```python
from build123d import *

# Parameters (mm, degrees)
SKETCH_1_R      = 1.6
SKETCH_1_R_2    = 7.25
EXTRUDE_1_DEPTH = 2
SKETCH_2_W      = 32.15
SKETCH_2_H      = 18.7
SKETCH_2_R      = 1.6
EXTRUDE_2_DEPTH = 2
FILLET_1_R      = 12
FILLET_2_R      = 1


with BuildPart() as part:
    # 草图1 → 凸台-拉伸1 (new body)
    with BuildSketch(Plane(origin=(0, 0, 0), x_dir=(1, 0, 0), z_dir=(0, 1, 0))):
        with BuildLine():
            Line((0, 0), (64.3, 0))
            Line((64.3, 0), (64.3, 30.6))
            ThreePointArc((64.3, 30.6), (60.521677477, 39.721677477), (51.4, 43.5))
            Line((51.4, 43.5), (12.9, 43.5))
            ThreePointArc((12.9, 43.5), (3.778322523, 39.721677477), (0, 30.6))
            Line((0, 30.6), (0, 0))
        make_face()
        with Locations(Location((7.89764523, 11.4, 0), (0, 0, 270))):
            Circle(SKETCH_1_R, mode=Mode.SUBTRACT)
        with Locations(Location((7.89764523, 37.8, 0), (0, 0, 270))):
            Circle(SKETCH_1_R, mode=Mode.SUBTRACT)
        with Locations(Location((12.9, 24.6, 0), (0, 0, 270))):
            Circle(SKETCH_1_R_2, mode=Mode.SUBTRACT)
        with Locations(Location((56.40235477, 11.4, 0), (0, 0, 90))):
            Circle(SKETCH_1_R, mode=Mode.SUBTRACT)
        with Locations(Location((56.40235477, 37.8, 0), (0, 0, 90))):
            Circle(SKETCH_1_R, mode=Mode.SUBTRACT)
        with Locations(Location((51.4, 24.6, 0), (0, 0, 90))):
            Circle(SKETCH_1_R_2, mode=Mode.SUBTRACT)
    extrude(amount=EXTRUDE_1_DEPTH)

    # 草图2 → 凸台-拉伸2 (add)
    # profile 1 of 2: a face of its own
    with BuildSketch(Plane.XY):
        with Locations((16.075, 11.35)):
            Rectangle(SKETCH_2_W, SKETCH_2_H)
        with Locations((3.15, 9.2)):
            Circle(SKETCH_2_R, mode=Mode.SUBTRACT)
        with Locations((17.15, 17.2)):
            Circle(SKETCH_2_R, mode=Mode.SUBTRACT)
    # profile 2 of 2: a face of its own
    with BuildSketch(Plane.XY):
        with Locations((48.225, 11.35)):
            Rectangle(SKETCH_2_W, SKETCH_2_H)
        with Locations((61.15, 9.2)):
            Circle(SKETCH_2_R, mode=Mode.SUBTRACT)
        with Locations((47.15, 17.2)):
            Circle(SKETCH_2_R, mode=Mode.SUBTRACT)
    extrude(amount=-EXTRUDE_2_DEPTH)

    # 圆角1
    fillet_1_edges = [part.edges().sort_by_distance(p)[0] for p in [
        (0, 20.7, -1),
        (64.3, 20.7, -1),
    ]]
    fillet(fillet_1_edges, radius=FILLET_1_R)

    # 圆角2
    fillet_2_edges = [part.edges().sort_by_distance(p)[0] for p in [
        (32.15, 2, -2),
        (32.15, 0, 0),
    ]]
    fillet(fillet_2_edges, radius=FILLET_2_R)


solid = part.part
```
Part model, mm, in its own coordinate system. A direction names the side the tool comes from. Round coordinates to 2 decimals unless told otherwise and drop trailing zeros. Write each loop counter-clockwise with the first axis right and the second up, starting at its lowest first coordinate (ties: lowest second). Pieces come first, ordered by that corner, then holes. Notation, with made-up numbers: M -10,-15.5 L -5,-15.5 A4 ccw -5,-9.5 Z; hole C 55.25,-34.75 d11. An arc over 180 degrees is marked long. Answer as CSV lines item,"result". Start each with the question number.
1) Mould opens along Z. For faces 3 (the face through (59.55, 9.27, -0.99)), 4 (the face through (32, 1, -43.5)), 5 (the face through (54.816, 0.986, -11.192)), 6 (the face through (7.97, 0.99, -39.4)) say: +Z half, -Z half, draft (parallel to the pull), parting line (faces both ways), or undercut.
2) Band-saw the part on B-B (x = 50). List the corners of the cut face in (y, z), then the cut area to 3 significant figures.
3) Band-saw the part on C-C (x = 17.15). List the corners of the cut face in (y, z), then the cut area to 3 significant figures.
4) Drop flat-ended pins along their axis: pin 1 (5 mm diameter, centred on x = 7.9, z = -11.4, fed in from +Y); pin 2 (3.5 mm diameter, centred on x = 17.15, y = 17.2, fed in from -Z). Give the stop position or say it passes through.
5) Which spindle directions (+Z, -Z, +X, -X, +Y, -Y) get a long thin tool onto all of the face, cutting with end or side? Do faces 1 (the face through (32, 12, -2)), 2 (the face through (3.42, 17.09, -1.01)). Say none if no direction does.
6) Band-saw the part on D-D (x = 39). List the corners of the cut face in (y, z), then the cut area to 3 significant figures.
7) Band-saw the part on A-A (z = -24.6). List the corners of the cut face in (x, y), then the cut area to 3 significant figures.
8) Drill centre lines: L1, parallel to X at y = 0.7, z = -24.6; L2, parallel to Y at x = 43.5, z = -9; L3, parallel to Z at x = 32, y = 13.5. Where is each one in solid material? Low to high.
Worked out:
1,face 3,"draft"
1,face 4,"-Z half"
1,face 5,"undercut"
1,face 6,"undercut"
2,outline,"M 0,-43.5 L 2,-43.5 L 2,-31.71 L 0,-31.71 Z; M 0,-17.49 L 2,-17.49 L 2,-3 A1 cw 3,-2 L 20.7,-2 L 20.7,0 L 1,0 A1 ccw 0,-1 Z"
2,area,"95.9 mm²"
3,outline,"M 0,-43.5 L 2,-43.5 L 2,-30.47 L 0,-30.47 Z; M 0,-18.73 L 2,-18.73 L 2,-3 A1 cw 3,-2 L 15.6,-2 L 15.6,0 L 1,0 A1 ccw 0,-1 Z; M 18.8,-2 L 20.7,-2 L 20.7,0 L 18.8,0 Z"
3,area,"94.5 mm²"
4,pin 1,"y = 2"
4,pin 2,"z = -2"
5,face 1,"-Z, +X, -X, +Y"
5,face 2,"+Z, -Z, -X, +Y"
6,outline,"M 0,-43.5 L 2,-43.5 L 2,-3 A1 cw 3,-2 L 20.7,-2 L 20.7,0 L 1,0 A1 ccw 0,-1 Z"
6,area,"124 mm²"
7,outline,"M 0,0 L 5.65,0 L 5.65,2 L 0,2 Z; M 20.15,0 L 44.15,0 L 44.15,2 L 20.15,2 Z; M 58.65,0 L 64.3,0 L 64.3,2 L 58.65,2 Z"
7,area,"70.6 mm²"
8,L1,"0 to 5.65, 20.15 to 44.15, 58.65 to 64.3"
8,L2,"0 to 2"
8,L3,"-2 to 0"
